Input: dimensioned drawing with shaded views. Units: mm. Origin: part minimum x, y, z. A direction names the side the tool comes from. Round coordinates to 2 decimals unless told otherwise and drop trailing zeros. Loops run counter-clockwise (first coordinate to the right, second up) from the corner with the lowest first, then second, coordinate; pieces in that order, holes last.
Item 1: Ray query, L1, parallel to Y at x = 4.15, z = 3.3; L2, parallel to X at y = 7, z = 2.3; L3, parallel to X at y = 5, z = 2.2. Return the intervals inside material, ascending.
Item 2: Section query C-C on y = 5.25. Return loops of the section in (x, z).
Item 3: Access query for the marked faces 1, 2 and 3. Directions: +Z, -Z, +X, -X, +Y, -Y. A direction counts if a zero-diameter tool reaches every point of the face in a straight line with its end or side. Return the directions, or none.
Item 4: Section query B-B on x = 2.7. Return loops of the section in (y, z), then the cut area to 3 significant figures.
Item 5: Section query D-D on z = 0.6. Return loops of the section in (x, y).
Item 6: Section query A-A on z = 1.95. Return loops of the section in (x, y).
Item 7: First-contact query: P1, Ø1.5, axis at x = 3.5, y = 1.5, coming from the +Z side; P2, Ø1, axis at x = 3.5, y = 6, coming from the -Z side. Flat tips, straight axial feed; report the tip coordinate or a pass-through.
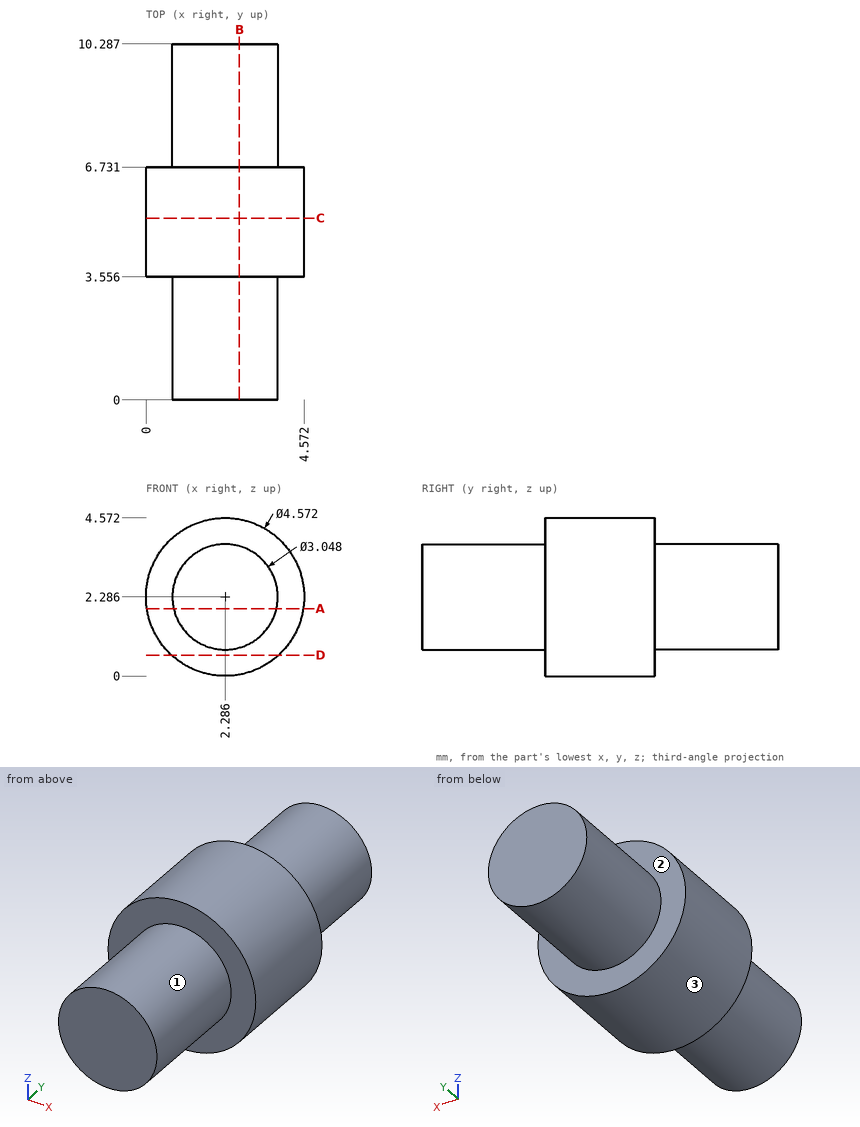
Data:
1. L1: y = 3.56 to 6.73
1. L2: x = 0.76 to 3.81
1. L3: x = 0 to 4.57
2. outline: circle Ø4.57 at (2.29, 2.29)
3. face 1: -Y
3. face 2: +Y
3. face 3: +Y, -Y
4. outline: (0, 0.82) - (3.56, 0.82) - (3.56, 0.04) - (6.73, 0.04) - (6.73, 0.82) - (10.29, 0.82) - (10.29, 3.75) - (6.73, 3.75) - (6.73, 4.53) - (3.56, 4.53) - (3.56, 3.75) - (0, 3.75) - close
4. area: 35.1 mm2
5. outline: (0.74, 3.56) - (3.83, 3.56) - (3.83, 6.73) - (0.74, 6.73) - close
6. outline: (0.02, 3.56) - (0.8, 3.56) - (0.8, 0) - (3.77, 0) - (3.77, 3.56) - (4.55, 3.56) - (4.55, 6.73) - (3.77, 6.73) - (3.77, 10.29) - (0.8, 10.29) - (0.8, 6.73) - (0.02, 6.73) - close
7. P1: stops at z = 3.74
7. P2: stops at z = 0.11
